Read the model definition and answer for the solid it produces. Units are mm, in the model's axes. Round coordinates to 2 decimals unless told otherwise and drop trailing zeros. Use one line per item in the form item = value. Start each with the question number.
1) The part is cut by section A-A, the plane x = 67. Count the separate pieces of the cut face and the enclosed holes in it, plus the area to 3 significant figures.
2) This flat-tipped pin is pushed along its axis until it touches: pin 1 (1.2 mm diameter, centred on x = 48.5, z = -10.5, fed in from +Y). Where does it stop, or does it pass through?
3) Consider line 1 along Y through (x, z) = (-147.5, -1.75); line 2 along Y through (x, z) = (-1.5, -13.9); line 3 along Z through (x, y) = (234.5, 12.6). Determine where each line is inside the solid, lowest interval first. Write a range as from..to.
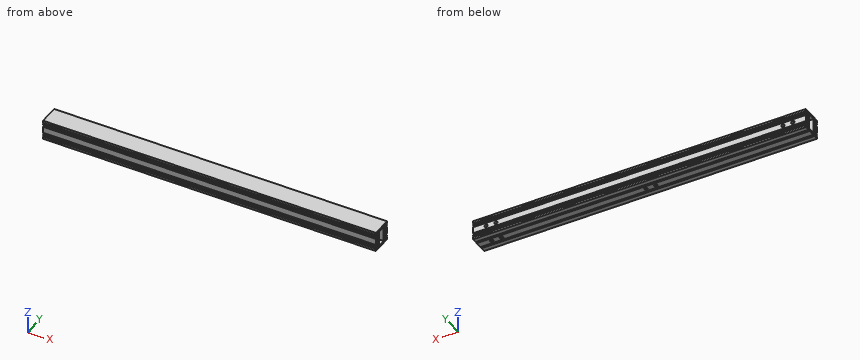
from build123d import *

# Parameters (mm, degrees)
SKETCH_1_W             = 23.5
SKETCH_1_H             = 12
EXTRUDE_1_DEPTH        = 254.5
HOLE_WIZARD_M6_1_D     = 5
HOLE_WIZARD_M6_1_DEPTH = 19
HOLE_WIZARD_M6_1_TIP   = 1.502151548
HOLE_WIZARD_M6_2_D     = 5
HOLE_WIZARD_M6_2_DEPTH = 19
HOLE_WIZARD_M6_2_TIP   = 1.502151548


with BuildPart() as part:
    # 草图1 → 凸台-拉伸1 (new, symmetric)
    with BuildSketch(Plane(origin=(0, 0, 0), x_dir=(0, 0, -1), z_dir=(1, 0, 0))):
        Polygon((-15, 15), (-11.5, 15), (-11.5, 13.5), (-11, 13.5), (-11, 12), (-9.5, 12), (-9.5, 15), (-8, 15), (-8, 12.5), (-5, 12.5), (-5, 15), (5, 15), (5, 12.5), (8, 12.5), (8, 15), (9.5, 15), (9.5, 12), (11, 12), (11, 13.5), (11.5, 13.5), (11.5, 15), (15, 15), (15, 8), (12.5, 8), (12.5, 5), (15, 5), (15, -5), (12.5, -5), (12.5, -8), (15, -8), (15, -15), (11.5, -15), (11.5, -13.5), (11, -13.5), (11, -12), (9.5, -12), (9.5, -15), (8, -15), (8, -12.5), (5, -12.5), (5, -15), (-5, -15), (-5, -12.5), (-8, -12.5), (-8, -15), (-9.5, -15), (-9.5, -12), (-11, -12), (-11, -13.5), (-11.5, -13.5), (-11.5, -15), (-15, -15), align=None)
        with BuildLine():
            Line((12, -10.5), (12, -8.5))
            ThreePointArc((12, -8.5), (11.853553391, -8.146446609), (11.5, -8))
            Line((11.5, -8), (-11.5, -8))
            ThreePointArc((-11.5, -8), (-11.853553391, -8.146446609), (-12, -8.5))
            Line((-12, -8.5), (-12, -10.5))
            ThreePointArc((-12, -10.5), (-11.853553391, -10.853553391), (-11.5, -11))
            Line((-11.5, -11), (11.5, -11))
            ThreePointArc((11.5, -11), (11.853553391, -10.853553391), (12, -10.5))
        make_face(mode=Mode.SUBTRACT)
        with BuildLine():
            Line((-11.5, 11), (11.5, 11))
            ThreePointArc((11.5, 11), (11.853553391, 10.853553391), (12, 10.5))
            Line((12, 10.5), (12, 8.5))
            ThreePointArc((12, 8.5), (11.853553391, 8.146446609), (11.5, 8))
            Line((11.5, 8), (-11.5, 8))
            ThreePointArc((-11.5, 8), (-11.853553391, 8.146446609), (-12, 8.5))
            Line((-12, 8.5), (-12, 10.5))
            ThreePointArc((-12, 10.5), (-11.853553391, 10.853553391), (-11.5, 11))
        make_face(mode=Mode.SUBTRACT)
        Rectangle(SKETCH_1_W, SKETCH_1_H, mode=Mode.SUBTRACT)
    extrude(amount=EXTRUDE_1_DEPTH, both=True)

    # M6 螺纹孔1
    with Locations(Plane(origin=(0, 0, -15), x_dir=(-1, 0, 0), z_dir=(0, 0, -1))):
        with Locations((-234.5, 0), (-219.5, 0), (1.5, 0), (16.5, 0)):
            Hole(HOLE_WIZARD_M6_1_D / 2, depth=HOLE_WIZARD_M6_1_DEPTH)
            with Locations((0, 0, -(HOLE_WIZARD_M6_1_DEPTH + HOLE_WIZARD_M6_1_TIP / 2))):  # 118° drill point
                Cone(0, HOLE_WIZARD_M6_1_D / 2, HOLE_WIZARD_M6_1_TIP, mode=Mode.SUBTRACT)

    # M6 螺纹孔2
    with Locations(Plane(origin=(0, 15, 0), x_dir=(1, 0, 0), z_dir=(0, 1, 0))):
        with Locations((234.5, 0), (219.5, 0), (-219.5, 0), (-234.5, 0)):
            Hole(HOLE_WIZARD_M6_2_D / 2, depth=HOLE_WIZARD_M6_2_DEPTH)
            with Locations((0, 0, -(HOLE_WIZARD_M6_2_DEPTH + HOLE_WIZARD_M6_2_TIP / 2))):  # 118° drill point
                Cone(0, HOLE_WIZARD_M6_2_D / 2, HOLE_WIZARD_M6_2_TIP, mode=Mode.SUBTRACT)


solid = part.part
Geometry results:
q1.separate_pieces = 1
q1.enclosed_holes = 3
q1.area = 408 mm2
q2.pin_1 = 13.5
q3.line_1 = -15..-11, -8..-6, 6..8, 11..15
q3.line_2 = -15..-8, -5..-2.5, 2.5..5, 8..15
q3.line_3 = -15..-11, -9.5..-8, -5..-2.5, 2.5..5, 8..9.5, 11..15
